Could you check a few things on this drawing? It's one solid part, dimensions in mm from its lowest x, y, z. A direction names the side the tool comes from. Round coordinates to 2 decimals unless told otherwise and drop trailing zeros. Write each loop counter-clockwise with the first axis right and the second up, starting at its lowest first coordinate (ties: lowest second). Pieces come first, ordered by that corner, then holes. Notation, with made-up numbers: (-26.5, 3) -> (31.5, 3) arc R34 ccw to (31.5, 41) -> close; hole circle Ø6 at (43.5, 81.5). An arc over 180 degrees is marked (long way). Answer in a Markdown table with one row per item. Add a question column.
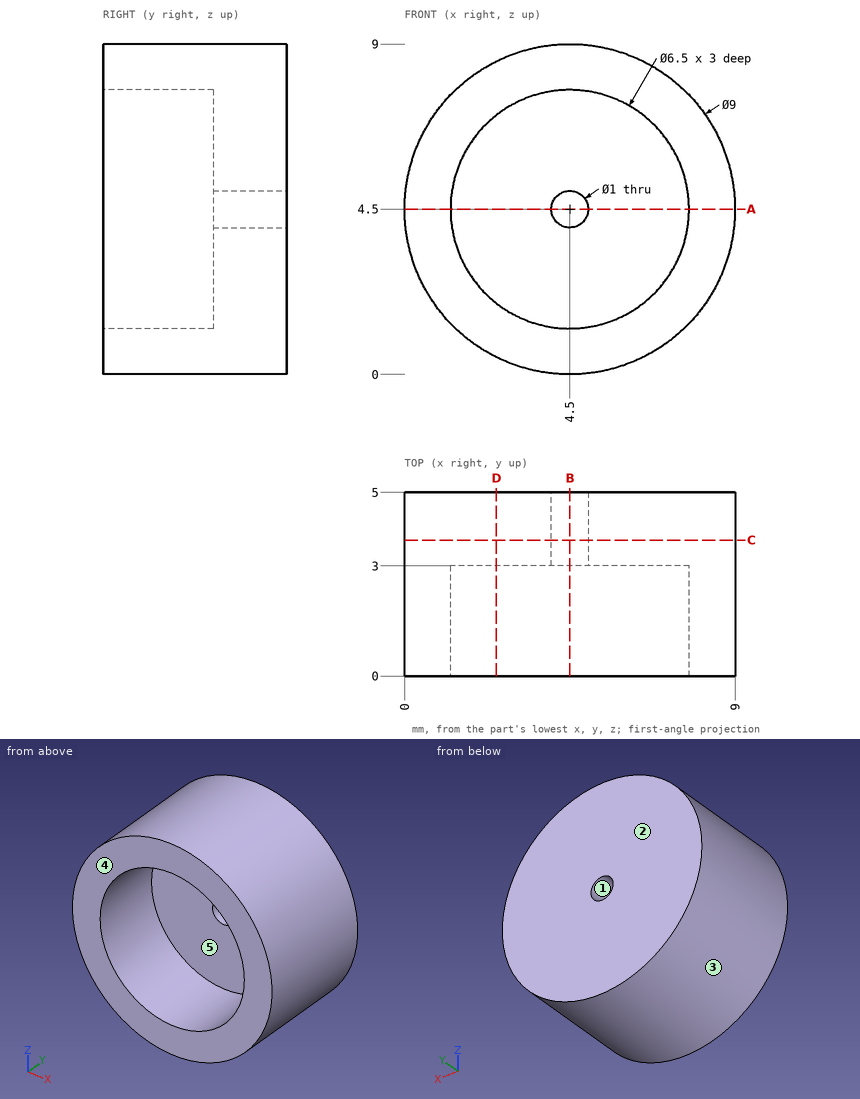
(1) Suppose I cut it at B-B, the plane x = 4.5. Please give me the cut outline in (y, z), then the cut area to 3 significant figures.
(2) On a 3-axis mill with a long thin cutter (end or side, diameter ignored), from which of +Z, -Z, +X, -X, +Y, -Y can I reach the whole of each face in a straight line? I mean the marked faces 4 and 5. Say none if no direction works.
(3) I need wall thicknesses on L1, parallel to Z at x = 4.5, y = 2.25; L2, parallel to Z at x = 4.5, y = 4; L3, parallel to X at y = 2.7, z = 4.25. Which ranges of each line are inside material? Lowest first, please.
(4) If we mould it in two halves opening along Z, with no side actions, what happens to the marked faces 1, 2 and 3? For each: pulls with the +Z half, pulls with the -Z half, needs draft (parallel to the pull), parting line crosses it, or undercut.
(5) Suppose I cut it at D-D, the plane x = 2.5. Please give me the cut outline in (y, z), then the cut area to 3 significant figures.
(6) For P1, Ø5, axis at x = 4.5, z = 4, coming from the -Y side, with a flat end and sliding along its axis, tell me the tip position at first contact or that it passes through.
(7) Suppose I cut it at C-C, the plane y = 3.7. Please give me the cut outline in (x, z).
(8) Suppose I cut it at A-A, the plane z = 4.5. Please give me the cut outline in (x, y), then the cut area to 3 significant figures.
Response:
| question | item | result |
|---|---|---|
| 1 | outline | (0, 0) -> (5, 0) -> (5, 4) -> (3, 4) -> (3, 1.25) -> (0, 1.25) -> close; (0, 7.75) -> (3, 7.75) -> (3, 5) -> (5, 5) -> (5, 9) -> (0, 9) -> close |
| 1 | area | 23.5 mm² |
| 2 | face 4 | +Z, -Z, +X, -X, -Y |
| 2 | face 5 | -Y |
| 3 | L1 | 0 to 1.25, 7.75 to 9 |
| 3 | L2 | 0 to 4, 5 to 9 |
| 3 | L3 | 0.01 to 1.26, 7.74 to 8.99 |
| 4 | face 1 | undercut |
| 4 | face 2 | needs draft |
| 4 | face 3 | parting line crosses it |
| 5 | outline | (0, 0.47) -> (5, 0.47) -> (5, 8.53) -> (0, 8.53) -> (0, 7.06) -> (3, 7.06) -> (3, 1.94) -> (0, 1.94) -> close |
| 5 | area | 24.9 mm² |
| 6 | P1 | y = 3 |
| 7 | outline | circle Ø9 at (4.5, 4.5); hole circle Ø1 at (4.5, 4.5) |
| 8 | outline | (0, 0) -> (1.25, 0) -> (1.25, 3) -> (4, 3) -> (4, 5) -> (0, 5) -> close; (5, 3) -> (7.75, 3) -> (7.75, 0) -> (9, 0) -> (9, 5) -> (5, 5) -> close |
| 8 | area | 23.5 mm² |
